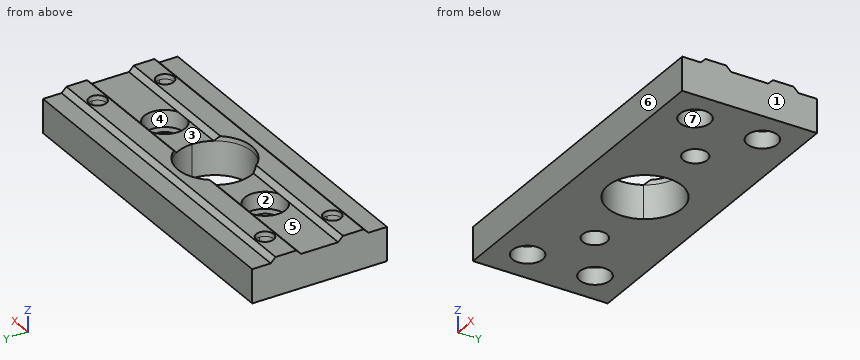
```python
from build123d import *
from build123d.topology import SkipClean

# Parameters (mm, degrees)
SKETCH1_W               = 100
SKETCH1_H               = 40
SKETCH1_R               = 11
SKETCH1_R_2             = 2.6
SKETCH1_R_3             = 3.6
BOSS_EXTRUDE1_DEPTH     = 10
CUT_EXTRUDE1_START      = 10
SKETCH2_R               = 6.05
CUT_EXTRUDE1_DEPTH      = 5
SKETCH3_R               = 4.5
CUT_EXTRUDE2_DEPTH      = 5
BOSS_EXTRUDE3_START     = -50
SKETCH4_W               = 1.43
SKETCH4_H               = 9
BOSS_EXTRUDE3_DEPTH     = 100
CHAMFER1_SIZE           = 1.43
CUT_EXTRUDE4_DEPTH      = 56.051293354
CUT_EXTRUDE4_DEPTH_BACK = 56.051293354
SKETCH5_R               = 11
SKETCH5_R_2             = 2.6


with BuildPart() as part:
    # Sketch1 → Boss-Extrude1 (new body)
    with BuildSketch(Plane.XY):
        Rectangle(SKETCH1_W, SKETCH1_H)
        Circle(SKETCH1_R, mode=Mode.SUBTRACT)
        with Locations((-40, 10)):
            Circle(SKETCH1_R_2, mode=Mode.SUBTRACT)
        with Locations((-40, -10)):
            Circle(SKETCH1_R_2, mode=Mode.SUBTRACT)
        with Locations((40, 10)):
            Circle(SKETCH1_R_2, mode=Mode.SUBTRACT)
        with Locations((40, -10)):
            Circle(SKETCH1_R_2, mode=Mode.SUBTRACT)
        with Locations((-24, 0)):
            Circle(SKETCH1_R_3, mode=Mode.SUBTRACT)
        with Locations((24, 0)):
            Circle(SKETCH1_R_3, mode=Mode.SUBTRACT)
    extrude(amount=BOSS_EXTRUDE1_DEPTH)

    # Sketch2 → Cut-Extrude1 (cut)
    with BuildSketch(Plane.XY.offset(CUT_EXTRUDE1_START)):
        with Locations(Location((24, 0, 0), (0, 0, 180))):
            Circle(SKETCH2_R)
        with Locations(Location((-24, 0, 0), (0, 0, 180))):
            Circle(SKETCH2_R)
    extrude(amount=-CUT_EXTRUDE1_DEPTH, mode=Mode.SUBTRACT)

    # Sketch3 → Cut-Extrude2 (cut)
    with BuildSketch(Plane.XY):
        with Locations((40, 10)):
            Circle(SKETCH3_R)
        with Locations((40, -10)):
            Circle(SKETCH3_R)
        with Locations((-40, 10)):
            Circle(SKETCH3_R)
        with Locations((-40, -10)):
            Circle(SKETCH3_R)
    extrude(amount=CUT_EXTRUDE2_DEPTH, mode=Mode.SUBTRACT)

    # Sketch4 → Boss-Extrude3 (add)
    with BuildSketch(Plane(origin=(0, 0, 0), x_dir=(0, 0, -1), z_dir=(1, 0, 0)).offset(BOSS_EXTRUDE3_START)):
        with Locations((-10.715, 10)):
            Rectangle(SKETCH4_W, SKETCH4_H)
        with Locations((-10.715, -10)):
            Rectangle(SKETCH4_W, SKETCH4_H)
    extrude(amount=BOSS_EXTRUDE3_DEPTH)

    # Chamfer1
    chamfer1_edges = [part.edges().sort_by_distance(p)[0] for p in [
        (0, -14.5, 11.43),
        (0, -5.5, 11.43),
        (0, 5.5, 11.43),
        (0, 14.5, 11.43),
    ]]
    chamfer(chamfer1_edges, length=CHAMFER1_SIZE - 0.0001)  # a hair under: the kernel refuses the full size

    # Sketch5 → Cut-Extrude4 (cut, two sides: drawn at the far end of the back side and taken through both)
    with SkipClean():  # the faces are left unmerged after this step: merging them gives an invalid solid
        with BuildSketch(Plane.XY.offset(-CUT_EXTRUDE4_DEPTH_BACK)):
            with Locations(Location((0, 0, 0), (0, 0, 150))):
                Circle(SKETCH5_R)
            with Locations(Location((-40, 10, 0), (0, 0, 180))):
                Circle(SKETCH5_R_2)
            with Locations(Location((-40, -10, 0), (0, 0, 180))):
                Circle(SKETCH5_R_2)
            with Locations(Location((40, -10, 0), (0, 0, 180))):
                Circle(SKETCH5_R_2)
            with Locations(Location((40, 10, 0), (0, 0, 180))):
                Circle(SKETCH5_R_2)
        extrude(amount=CUT_EXTRUDE4_DEPTH + CUT_EXTRUDE4_DEPTH_BACK, mode=Mode.SUBTRACT)


solid = part.part
```
The listing builds one solid part. Answer for the finished solid, in the listing's coordinates (mm). Face numbers are marked on the shaded views. A direction names the side the tool comes from. Give positions to 0.01 mm unless a question says otherwise; leave off trailing zeros. Loops run counter-clockwise (first coordinate to the right, second up) from the corner with the lowest first, then second, coordinate; pieces in that order, holes last. Notation, with made-up numbers: (-39, -8) - (-18, -8) arc R36 ccw to (-18, 29) - close; hole circle Ø2 at (50.5, 52). An arc over 180 degrees is marked (long way). Return JSON: item names as keys, results as strings. Group by question number.
1. Find section B-B (x = 40). State how many separate pieces and enclosed holes the cut face has, then the cut area to 3 significant figures.
2. Find section D-D (z = 3.5). Write down the section's boundary in (x, y), then the cut area to 3 significant figures.
3. Given pin 1 Ø4 at (x, y) = (40, -10) entering from -Z; pin 2 Ø3.5 at (x, y) = (-14.5, 2) entering from +Z; pin 3 Ø3.5 at (x, y) = (25, -2) entering from +Z; pin 4 Ø8 at (x, y) = (-40, -10) entering from -Z, each flat-ended and moving along its own axis, determine where each tip first touches the part or whether it passes through.
4. Which of the six approach directions +Z, -Z, +X, -X, +Y, -Y give full straight-line access (tool end or side, diameter ignored) to the marked faces 4, 5, 6 and 7?
5. Determine the mould class of the marked faces 1, 2 and 3 for opening direction X: pulls with the +X half, pulls with the -X half, needs draft (parallel to the pull), parting line crosses it, or undercut.
6. Find section C-C (y = 9). Write down the section's boundary in (x, z), then the cut area to 3 significant figures.
7. Straight lines are drawn through the part: line 1 (X direction, y = -0.5, z = 7.25); line 2 (Y direction, x = 24, z = 3.5); line 3 (X direction, y = -10, z = 10.55). For each, find the intervals that lie inside material, in ascending order. Write a range as [from, to].
Verdict:
{
 "1": {"separate pieces": "3", "enclosed holes": "0", "area": "265 mm^2"},
 "2": {"outline": "(-50, -20) - (50, -20) - (50, 20) - (-50, 20) - close; hole circle Ø9 at (-40, -10); hole circle Ø9 at (-40, 10); hole circle Ø7.2 at (-24, 0); hole circle Ø22 at (0, 0); hole circle Ø7.2 at (24, 0); hole circle Ø9 at (40, -10); hole circle Ø9 at (40, 10)", "area": "3,280 mm^2"},
 "3": {"pin 1": "passes through", "pin 2": "stops at z = 10", "pin 3": "stops at z = 5", "pin 4": "stops at z = 5"},
 "4": {"face 4": "none", "face 5": "+Z, +X, -X", "face 6": "+Z, -Z, +X, -X, -Y", "face 7": "-Z"},
 "5": {"face 1": "pulls with the +X half", "face 2": "undercut", "face 3": "needs draft"},
 "6": {"outline": "(-50, 0) - (-44.39, 0) - (-44.39, 5) - (-42.4, 5) - (-42.4, 11.43) - (-50, 11.43) - close; (-37.6, 5) - (-35.61, 5) - (-35.61, 0) - (-6.32, 0) - (-6.32, 11.43) - (-37.6, 11.43) - close; (6.32, 0) - (35.61, 0) - (35.61, 5) - (37.6, 5) - (37.6, 11.43) - (6.32, 11.43) - close; (42.4, 5) - (44.39, 5) - (44.39, 0) - (50, 0) - (50, 11.43) - (42.4, 11.43) - close", "area": "849 mm^2"},
 "7": {"line 1": "x = [-50, -30.03], [-17.97, -10.99], [10.99, 17.97], [30.03, 50]", "line 2": "y = [-20, -3.6], [3.6, 20]", "line 3": "x = [-50, -42.6], [-37.4, -4.58], [4.58, 37.4], [42.6, 50]"}
}
